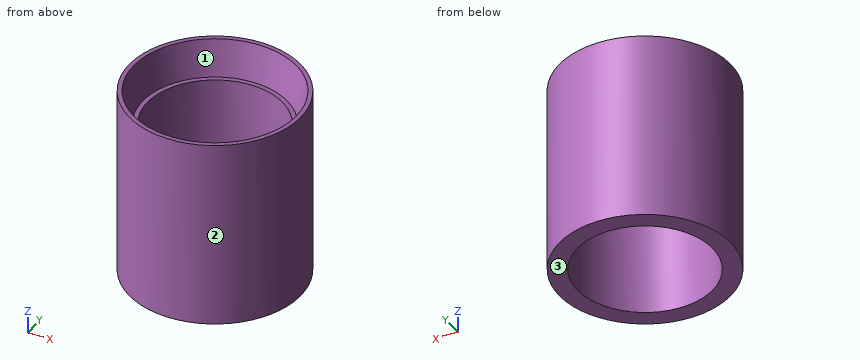
```python
from build123d import *

# Parameters (mm, degrees)
F0_R     = 31.75
F1_DEPTH = 69.85
F2_R     = 30.1625
F3_DEPTH = 12.7
F3_TAPER = 15
F4_R     = 25.0825
F5_DEPTH = 57.151


with BuildPart() as f1:
    # F0 (on Top) → F1 (new body)
    with BuildSketch(Plane.XY):
        Circle(F0_R)
    extrude(amount=F1_DEPTH)

    # F2 (on face) → F3 (cut)
    with BuildSketch(Plane.XY.offset(69.85)):
        Circle(F2_R)
    extrude(amount=-F3_DEPTH, taper=F3_TAPER, mode=Mode.SUBTRACT)

    # F4 (on face) → F5 (cut, through all)
    with BuildSketch(Plane.XY.offset(57.15)):
        Circle(F4_R)
    extrude(amount=-F5_DEPTH, mode=Mode.SUBTRACT)


solid = f1.part
```
The listing builds one solid part. Answer for the finished solid, in the listing's coordinates (mm). Face numbers are marked on the shaded views. Round coordinates to 2 decimals unless told otherwise and drop trailing zeros. Order: outer loops, then holes, each group sorted by start corner. A loop starts at its lowest first (then second) coordinate and runs counter-clockwise, first axis right, second up. Notation, with made-up numbers: (-0.5, 50.25) -> (36.5, 50.25) arc R29 cw to (36.5, 79.25) -> close; hole circle Ø3 at (80.25, -10.75). An arc over 180 degrees is marked (long way). Answer as CSV lines item,"result".
Q1. A cutting plane is placed at A-A on x = 0. Determine the outline of the cut face in (y, z).
Computed values:
outline,"(-31.75, 0) -> (-25.08, 0) -> (-25.08, 57.15) -> (-26.76, 57.15) -> (-30.16, 69.85) -> (-31.75, 69.85) -> close; (25.08, 0) -> (31.75, 0) -> (31.75, 69.85) -> (30.16, 69.85) -> (26.76, 57.15) -> (25.08, 57.15) -> close"
Q2. For a pull along Y with two mould halves and no side action, classify the marked faces 1, 2 and 3 as +Y half, -Y half, draft (parallel to the pull), parting line (faces both ways), or undercut.
Computed values:
face 1,"undercut"
face 2,"parting line"
face 3,"draft"
Q3. Consider line 1 (Y direction, x = 0, z = 25); line 2 (X direction, y = -1, z = 37); line 3 (Z direction, x = -26, y = 1). Determine where each line is inside the solid, lowest interval first. Write a range as from..to.
Computed values:
line 1,"y = -31.75..-25.08, 25.08..31.75"
line 2,"x = -31.73..-25.06, 25.06..31.73"
line 3,"z = 0..57.15"
Q4. Given pin 1 (1 mm diameter, centred on x = 4, z = 31, fed in from +Y); pin 2 (1.5 mm diameter, centred on y = -19, z = 41.5, fed in from +X); pin 3 (10 mm diameter, centred on x = 17.5, z = 47.5, fed in from -Y), each flat-ended and moving along its own axis, determine where each tip first touches the part or whether it passes through.
Computed values:
pin 1,"stops at y = 31.56"
pin 2,"stops at x = 25.98"
pin 3,"stops at y = -29.19"
